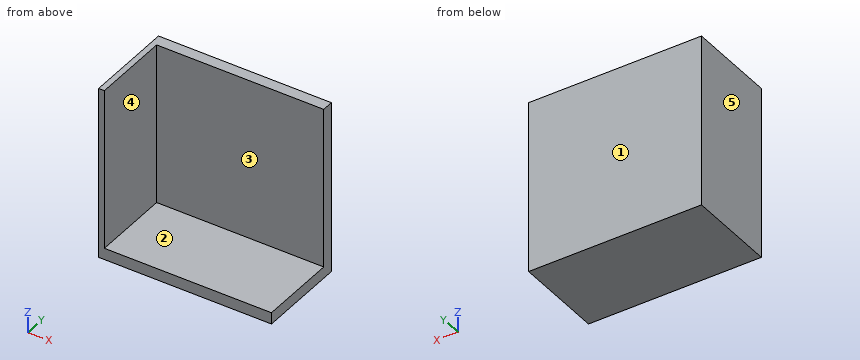
from build123d import *

# Parameters (mm, degrees)
F1_DEPTH = 90
F3_W     = 47
F3_H     = 90
F4_DEPTH = 3


# Not quite as in the source:
# - the program builds the solid bodies; features that only make, move or delete a surface that nothing else refers to are left out


with BuildPart() as f1:
    # F0 (on Right) → F1 (new body)
    with BuildSketch(Plane.YZ):
        Polygon((47, 0), (47, 90), (41, 90), (41, 6), (0, 6), (0, 0), align=None)
    extrude(amount=F1_DEPTH)

    # F3 (on face) → F4 (join)
    with BuildSketch(Plane(origin=(0, 0, 0), x_dir=(0, -1, 0), z_dir=(-1, 0, 0))):
        with Locations((-23.5, 45)):
            Rectangle(F3_W, F3_H)
    extrude(amount=-F4_DEPTH)


solid = f1.part
Source: CAD feature listing. Evaluate the final solid. Frame: model axes, mm. Face numbers are marked on the shaded views. A direction names the side the tool comes from. Give positions to 0.01 mm unless a question says otherwise; leave off trailing zeros. Write each loop counter-clockwise with the first axis right and the second up, starting at its lowest first coordinate (ties: lowest second). Pieces come first, ordered by that corner, then holes. Notation, with made-up numbers: M 59,62.5 L 97,62.5 A18 ccw 97,97.5 Z; hole C 67.5,55.25 d1. An arc over 180 degrees is marked long. Return JSON: item names as keys, results as strings. Group by question number.
1) Ray query, L1, parallel to X at y = 5, z = 32; L2, parallel to Z at x = 41.5, y = 15.5; L3, parallel to Y at x = 63.5, z = 61.5. Return the intervals inside material, ascending.
2) Draft query along Y for the marked faces 1, 2 and 3. Return one class per face: released by +Y, released by -Y, zero draft, split by the parting line, or undercut.
3) Cut plane B-B, the plane z = 66. Output: boundary loops of the cut face in (x, y).
4) First-contact query: pin 1 Ø20.5 at (x, y) = (39, 24.5) entering from +Z; pin 2 Ø3 at (x, z) = (61, 69) entering from -Y; pin 3 Ø12 at (y, z) = (6, 36) entering from +X. Flat tips, straight axial feed; report the tip coordinate or a pass-through.
5) Cut plane A-A, the plane x = 15. Output: boundary loops of the cut face in (y, z).
6) Set-up query: the marked faces 4 and 5. Return all of +Z, -Z, +X, -X, +Y, -Y with unobstructed straight access to the full face (end or side cutting, diameter ignored); none if empty.
Data:
{
 "1": {"L1": "x = 0 to 3", "L2": "z = 0 to 6", "L3": "y = 41 to 47"},
 "2": {"face 1": "released by +Y", "face 2": "zero draft", "face 3": "released by -Y"},
 "3": {"outline": "M 0,0 L 3,0 L 3,41 L 90,41 L 90,47 L 0,47 Z"},
 "4": {"pin 1": "stops at z = 6", "pin 2": "stops at y = 41", "pin 3": "stops at x = 3"},
 "5": {"outline": "M 0,0 L 47,0 L 47,90 L 41,90 L 41,6 L 0,6 Z"},
 "6": {"face 4": "+Z, +X, -Y", "face 5": "+Z, -Z, -X, +Y, -Y"}
}
